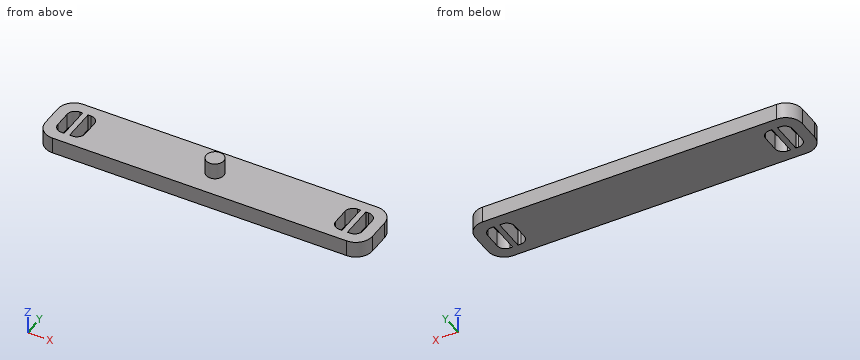
from build123d import *

# Parameters (mm, degrees)
SKETCH1_W           = 60
SKETCH1_H           = 10
BOSS_EXTRUDE1_DEPTH = 3
CUT_EXTRUDE2_DEPTH  = 3
FILLET1_R           = 3
SKETCH2_R           = 1.6
BOSS_EXTRUDE2_DEPTH = 3


with BuildPart() as part:
    # Sketch1 → Boss-Extrude1 (new body)
    with BuildSketch(Plane.XY):
        Rectangle(SKETCH1_W, SKETCH1_H)
    extrude(amount=BOSS_EXTRUDE1_DEPTH)

    # Sketch3 → Cut-Extrude2 (cut)
    with BuildSketch(Plane.XY.offset(3)):
        with BuildLine():
            Line((-26.5, 3), (-26, 3))
            Line((-26, 3), (-26, -3))
            Line((-26, -3), (-26.5, -3))
            ThreePointArc((-26.5, -3), (-27.560660172, -2.560660172), (-28, -1.5))
            Line((-28, -1.5), (-28, 1.5))
            ThreePointArc((-28, 1.5), (-27.560660172, 2.560660172), (-26.5, 3))
        make_face()
        with BuildLine():
            Line((-25, 3), (-24.5, 3))
            ThreePointArc((-24.5, 3), (-23.439339828, 2.560660172), (-23, 1.5))
            Line((-23, 1.5), (-23, -1.5))
            ThreePointArc((-23, -1.5), (-23.439339828, -2.560660172), (-24.5, -3))
            Line((-24.5, -3), (-25, -3))
            Line((-25, -3), (-25, 3))
        make_face()
    cut_extrude2 = extrude(amount=-CUT_EXTRUDE2_DEPTH, mode=Mode.SUBTRACT)

    # Mirror1: Cut-Extrude2 across plane
    add(cut_extrude2.mirror(Plane(origin=(0, 0, 0), x_dir=(0, 0, 1), z_dir=(1, 0, 0))), mode=Mode.SUBTRACT)

    # Fillet1
    fillet1_edges = [part.edges().sort_by_distance(p)[0] for p in [
        (30, -5, 1.5),
        (-30, -5, 1.5),
        (-30, 5, 1.5),
        (30, 5, 1.5),
    ]]
    fillet(fillet1_edges, radius=FILLET1_R)

    # Sketch2 → Boss-Extrude2 (add)
    with BuildSketch(Plane.XY.offset(3)):
        Circle(SKETCH2_R)
    extrude(amount=BOSS_EXTRUDE2_DEPTH)


solid = part.part
Input: part model. Units: mm. Frame: model coordinates. Give positions to 0.01 mm unless a question says otherwise; leave off trailing zeros. Write each loop counter-clockwise with the first axis right and the second up, starting at its lowest first coordinate (ties: lowest second). Pieces come first, ordered by that corner, then holes.
Q1. Section B-B, the plane x = 0. Output: boundary loops of the cut face in (y, z), plus the area to 3 significant figures.
Q2. First-contact query: P1, Ø1.5, axis at x = 19.5, y = 3, coming from the -Z side; P2, Ø3, axis at x = 16, y = -1.5, coming from the +Z side; P3, Ø1.5, axis at y = 3, z = 5.5, coming from the -X side. Flat tips, straight axial feed; report the tip coordinate or a pass-through.
Q3. Section C-C, the plane z = 2.1. State how many separate pieces and enclosed holes the cut face has, plus the area to 3 significant figures.
Q4. Material intervals for probe 1 along X at (y, z) = (-0.75, 2.05); probe 2 along Y at (x, z) = (-26.5, 2.6); probe 3 along X at (y, z) = (-2.5, 2.9), sorted ascending.
Q5. Section D-D, the plane z = 5.15. Output: boundary loops of the cut face in (x, y), plus the area to 3 significant figures.
Q6. Section A-A, the plane y = 0. Output: boundary loops of the cut face in (x, z).
Filled in:
1. outline: (-5, 0) - (5, 0) - (5, 3) - (1.6, 3) - (1.6, 6) - (-1.6, 6) - (-1.6, 3) - (-5, 3) - close
1. area: 39.6 mm2
2. P1: stops at z = 0
2. P2: stops at z = 3
2. P3: passes through
3. separate pieces: 1
3. enclosed holes: 4
3. area: 548 mm2
4. probe 1: x = -30 to -28, -26 to -25, -23 to 23, 25 to 26, 28 to 30
4. probe 2: y = -5 to -3, 3 to 5
4. probe 3: x = -29.96 to -27.62, -26 to -25, -23.38 to 23.38, 25 to 26, 27.62 to 29.96
5. outline: circle Ø3.2 at (0, 0)
5. area: 8.04 mm2
6. outline: (-30, 0) - (-28, 0) - (-28, 3) - (-30, 3) - close; (-26, 0) - (-25, 0) - (-25, 3) - (-26, 3) - close; (-23, 0) - (23, 0) - (23, 3) - (1.6, 3) - (1.6, 6) - (-1.6, 6) - (-1.6, 3) - (-23, 3) - close; (25, 0) - (26, 0) - (26, 3) - (25, 3) - close; (28, 0) - (30, 0) - (30, 3) - (28, 3) - close
